Verification items for the finished model (mm, model axes). A direction names the side the tool comes from. Coordinates: 2 decimals unless noted, no trailing zeros. Order: outer loops, then holes, each group sorted by start corner. A loop starts at its lowest first (then second) coordinate and runs counter-clockwise, first axis right, second up. Notation, with made-up numbers: M 13,68.25 L 40,68.25 A26 cw 40,103.25 Z; hole C -34.5,-3 d1. An arc over 180 degrees is marked long. Return JSON: item names as keys, results as strings. Group by question number.
1. Gauge pin test, flat ends, axial feed: pin 1 (7 mm diameter, centred on x = 35, z = -10, fed in from +Y); pin 2 (6 mm diameter, centred on y = 9.5, z = 7, fed in from -X); pin 3 (1.6 mm diameter, centred on x = 19, z = -8.5, fed in from -Y); pin 4 (3 mm diameter, centred on x = 28, z = 20, fed in from -Y). Record the tip position at first contact, or that the pin passes through.
2. Section check D-D, the plane z = -10. Record the cut outline in (x, y).
3. Material ranges on line 1 along X through (y, z) = (36, 12); line 2 along Z through (x, y) = (24, 35); line 3 along Z through (x, y) = (23.5, 10), recorded low to high.
4. Section check C-C, the plane z = 1.5. Record the cut outline in (x, y).
5. Section check A-A, the plane y = 10. Record the cut outline in (x, z).
6. Mould release check, pull along X, two halves, no side actions. Record for faces 1 (the flat face through (32, 16, 0)), 2 (the flat face through (45, 19, -10)), 3 (the cylindrical face through (9.19, 34.34, 4.01)): +X half, -X half, draft (parallel to the pull), parting line (faces both ways), or undercut.
7. Set-up check for faces 4 (the flat face through (20, 32, -4)), 5 (the flat face through (33, 10, 5)), 6 (the flat face through (31, 20, 12)), 7 (the flat face through (10, 33, 5)): record each of +Z, -Z, +X, -X, +Y, -Y from which the full face is reachable in a straight line by a thin tool's end or side.
```python
from build123d import *

# Parameters (mm, degrees)
F1_DEPTH  = 5
F3_DEPTH  = 25
F4_DEPTH  = 25
F6_DEPTH  = 45.001
F7_W      = 27
F7_H      = 5.42
F7_W_2    = 5.42
F7_H_2    = 27
F8_DEPTH  = 2
F10_DEPTH = 45.001
F12_DEPTH = 30
F13_R     = 2.25
F14_DEPTH = 7.001
F15_R     = 2.25
F16_DEPTH = 25.001
F17_R     = 2.25
F18_DEPTH = 25.001
F20_DEPTH = 20
F22_DEPTH = 2
F23_W     = 27
F23_H     = 5.42
F24_DEPTH = 2
F25_R     = 2.25
F26_DEPTH = 25.001
F27_R     = 2.25
F28_DEPTH = 25.001
F29_R     = 3.75
F30_DEPTH = 2
F31_R     = 3.75
F32_DEPTH = 2
F33_R     = 3.75
F34_DEPTH = 2
F35_R     = 3.75
F36_DEPTH = 2
F37_R     = 3.75
F38_DEPTH = 2
F39_R     = 3.75
F40_DEPTH = 2
F41_W     = 2
F41_H     = 2
F42_DEPTH = 12.711
F43_W     = 2
F43_H     = 2
F44_DEPTH = 12.711
F45_W     = 2
F45_H     = 2
F46_DEPTH = 12.711


with BuildPart() as f1:
    # F0 (on Top) → F1 (new body)
    with BuildSketch(Plane.XY):
        Polygon((0, 20), (20, 20), (20, 0), (45, 0), (45, 20), (20, 45), (0, 45), align=None)
    extrude(amount=F1_DEPTH)

    # F2 (on face) → F3 (join)
    with BuildSketch(Plane.XY.offset(5)):
        Polygon((0, 25), (0, 20), (20, 20), (20, 0), (25, 0), (45, 0), (45, 5), (25, 5), (25, 15), (45, 15), (45, 20), (25, 20), (20, 25), (20, 45), (15, 45), (15, 25), (5, 25), (5, 45), (0, 45), align=None)
    extrude(amount=F3_DEPTH)

    # F2 (on face) → F4 (join)
    with BuildSketch(Plane.XY.offset(5)):
        Polygon((0, 25), (0, 20), (20, 20), (20, 0), (25, 0), (45, 0), (45, 5), (25, 5), (25, 15), (45, 15), (45, 20), (25, 20), (20, 25), (20, 45), (15, 45), (15, 25), (5, 25), (5, 45), (0, 45), align=None)
    extrude(amount=F4_DEPTH)

    # F5 (on face) → F6 (cut, through all)
    with BuildSketch(Plane(origin=(0, 0, 0), x_dir=(0, -1, 0), z_dir=(-1, 0, 0))):
        Polygon((-45, 30), (-45, 5), (-25, 30), align=None)
    extrude(amount=-F6_DEPTH, mode=Mode.SUBTRACT)

    # F7 (on face) → F8 (join)
    with BuildSketch(Plane(origin=(0, 0, 0), x_dir=(1, 0, 0), z_dir=(0, 0, -1))):
        with Locations((31.5, -10)):
            Rectangle(F7_W, F7_H)
        with Locations((10, -31.5)):
            Rectangle(F7_W_2, F7_H_2)
    extrude(amount=F8_DEPTH)

    # F9 (on face) → F10 (cut, through all)
    with BuildSketch(Plane.XZ):
        Polygon((45, 30), (25, 30), (45, 5), align=None)
    extrude(amount=-F10_DEPTH, mode=Mode.SUBTRACT)

    # F11 (on face) → F12 (join)
    with BuildSketch(Plane.XY.offset(30)):
        Polygon((12.71, 20), (10, 20), (7.29, 20), (7.29, 18), (12.71, 18), align=None)
        Polygon((20, 7.29), (20, 10), (20, 12.71), (18, 12.71), (18, 7.29), align=None)
    extrude(amount=-F12_DEPTH)

    # F13 (on face) → F14 (cut, through all)
    with BuildSketch(Plane.XY.offset(5)):
        with Locations((10, 38)):
            Circle(F13_R)
        with Locations((38, 10)):
            Circle(F13_R)
    extrude(amount=-F14_DEPTH, mode=Mode.SUBTRACT)

    # F15 (on face) → F16 (cut, through all)
    with BuildSketch(Plane(origin=(0, 25, 0), x_dir=(-1, 0, 0), z_dir=(0, 1, 0))):
        with Locations((-10, 23)):
            Circle(F15_R)
    extrude(amount=-F16_DEPTH, mode=Mode.SUBTRACT)

    # F17 (on face) → F18 (cut, through all)
    with BuildSketch(Plane.YZ.offset(25)):
        with Locations((10, 23)):
            Circle(F17_R)
    extrude(amount=-F18_DEPTH, mode=Mode.SUBTRACT)

    # F19 (on face) → F20 (join)
    with BuildSketch(Plane(origin=(0, 0, 0), x_dir=(1, 0, 0), z_dir=(0, 0, -1))):
        Polygon((40, -25), (45, -20), (20, -20), (20, -45), (25, -40), (25, -25), align=None)
    extrude(amount=F20_DEPTH)

    # F21 (on face) → F22 (join)
    with BuildSketch(Plane.XZ.offset(-20)):
        Polygon((45, -12.71), (45, -10), (45, -7.29), (20, -7.29), (20, -12.71), align=None)
    extrude(amount=F22_DEPTH)

    # F23 (on face) → F24 (join)
    with BuildSketch(Plane(origin=(20, 0, 0), x_dir=(0, -1, 0), z_dir=(-1, 0, 0))):
        with Locations((-31.5, -10)):
            Rectangle(F23_W, F23_H)
    extrude(amount=F24_DEPTH)

    # F25 (on face) → F26 (cut, through all)
    with BuildSketch(Plane.YZ.offset(25)):
        with Locations((35, -10)):
            Circle(F25_R)
    extrude(amount=-F26_DEPTH, mode=Mode.SUBTRACT)

    # F27 (on face) → F28 (cut, through all)
    with BuildSketch(Plane(origin=(0, 25, 0), x_dir=(-1, 0, 0), z_dir=(0, 1, 0))):
        with Locations((-35, -10)):
            Circle(F27_R)
    extrude(amount=-F28_DEPTH, mode=Mode.SUBTRACT)

    # F29 (on face) → F30 (cut)
    with BuildSketch(Plane(origin=(0, 25, 0), x_dir=(-1, 0, 0), z_dir=(0, 1, 0))):
        with Locations((-35, -10)):
            Circle(F29_R)
    extrude(amount=-F30_DEPTH, mode=Mode.SUBTRACT)

    # F31 (on face) → F32 (cut)
    with BuildSketch(Plane.YZ.offset(25)):
        with Locations((35, -10)):
            Circle(F31_R)
    extrude(amount=-F32_DEPTH, mode=Mode.SUBTRACT)

    # F33 (on face) → F34 (cut)
    with BuildSketch(Plane(origin=(0, 25, 0), x_dir=(-1, 0, 0), z_dir=(0, 1, 0))):
        with Locations((-10, 23)):
            Circle(F33_R)
    extrude(amount=-F34_DEPTH, mode=Mode.SUBTRACT)

    # F35 (on face) → F36 (cut)
    with BuildSketch(Plane.YZ.offset(25)):
        with Locations((10, 23)):
            Circle(F35_R)
    extrude(amount=-F36_DEPTH, mode=Mode.SUBTRACT)

    # F37 (on face) → F38 (cut)
    with BuildSketch(Plane.XY.offset(5)):
        with Locations((38, 10)):
            Circle(F37_R)
    extrude(amount=-F38_DEPTH, mode=Mode.SUBTRACT)

    # F39 (on face) → F40 (cut)
    with BuildSketch(Plane.XY.offset(5)):
        with Locations((10, 38)):
            Circle(F39_R)
    extrude(amount=-F40_DEPTH, mode=Mode.SUBTRACT)

    # F41 (on face) → F42 (cut, through all)
    with BuildSketch(Plane.XY.offset(-7.29)):
        with Locations((19, 19)):
            Rectangle(F41_W, F41_H)
    extrude(amount=-F42_DEPTH, mode=Mode.SUBTRACT)

    # F43 (on face) → F44 (cut, through all)
    with BuildSketch(Plane.YZ.offset(12.71)):
        with Locations((19, -1)):
            Rectangle(F43_W, F43_H)
    extrude(amount=-F44_DEPTH, mode=Mode.SUBTRACT)

    # F45 (on face) → F46 (cut, through all)
    with BuildSketch(Plane(origin=(0, 12.71, 0), x_dir=(-1, 0, 0), z_dir=(0, 1, 0))):
        with Locations((-19, -1)):
            Rectangle(F45_W, F45_H)
    extrude(amount=-F46_DEPTH, mode=Mode.SUBTRACT)


solid = f1.part
```
Answers follow:
{
 "1": {"pin 1": "y = 23", "pin 2": "x = 18", "pin 3": "y = 20", "pin 4": "y = 0"},
 "2": {"outline": "M 18,20 L 20,20 L 20,18 L 32.75,18 L 32.75,23 L 31.25,23 L 31.25,25 L 25,25 L 25,31.25 L 23,31.25 L 23,32.75 L 18,32.75 Z; M 18,37.25 L 23,37.25 L 23,38.75 L 25,38.75 L 25,40 L 20,45 L 18,45 Z; M 37.25,18 L 45,18 L 45,20 L 40,25 L 38.75,25 L 38.75,23 L 37.25,23 Z"},
 "3": {"line 1": "0 to 5, 15 to 20", "line 2": "-20 to -13.75, -6.25 to 5", "line 3": "-2 to 19.25, 26.75 to 30"},
 "4": {"outline": "M 0,20 L 7.29,20 L 7.29,18 L 12.71,18 L 12.71,20 L 20,20 L 20,12.71 L 18,12.71 L 18,7.29 L 20,7.29 L 20,0 L 45,0 L 45,20 L 20,45 L 0,45 Z; hole C 10,38 d4.5; hole C 38,10 d4.5"},
 "5": {"outline": "M 18,0 L 20,0 L 20,-2 L 35.75,-2 L 35.75,3 L 34.25,3 L 34.25,5 L 25,5 L 25,19.25 L 23,19.25 L 23,20.75 L 18,20.75 Z; M 18,25.25 L 23,25.25 L 23,26.75 L 25,26.75 L 25,30 L 18,30 Z; M 40.25,-2 L 45,-2 L 45,5 L 41.75,5 L 41.75,3 L 40.25,3 Z"},
 "6": {"face 1": "draft", "face 2": "+X half", "face 3": "undercut"},
 "7": {"face 4": "+Y, -Y", "face 5": "+Z, +X", "face 6": "+Z, +X, +Y", "face 7": "+Z, +Y"}
}
